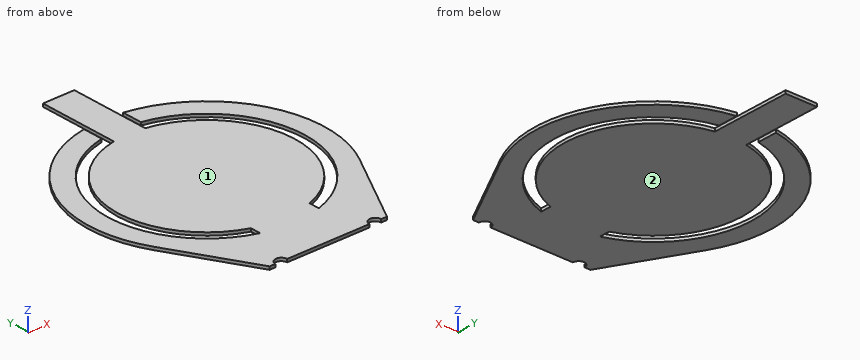
```python
from build123d import *

# Parameters (mm, degrees)
BOSS_EXTRUDE1_DEPTH      = 0.75438
CORTE_EXTRUS_O1_START    = -10
CORTE_EXTRUS_O1_DEPTH    = 10
RESSALTO_EXTRUS_O1_START = -0.75438
RESSALTO_EXTRUS_O1_DEPTH = 0.75438
CORTE_EXTRUS_O2_DEPTH    = 10


with BuildPart() as part:
    # Sketch1 → Boss-Extrude1 (new body)
    with BuildSketch(Plane.XY):
        with BuildLine():
            Line((-15, -35), (15, -35))
            Line((15, -35), (26.292884648, -14.44590658))
            ThreePointArc((26.292884648, -14.44590658), (0, 30), (-26.292884648, -14.44590658))
            Line((-26.292884648, -14.44590658), (-15, -35))
        make_face()
        with BuildLine():
            Line((-7.5, -23.848480035), (-7.5, -21.213203436))
            ThreePointArc((-7.5, -21.213203436), (0, 22.5), (7.5, -21.213203436))
            Line((7.5, -21.213203436), (7.5, -23.848480035))
            ThreePointArc((7.5, -23.848480035), (0, 25), (-7.5, -23.848480035))
        make_face(mode=Mode.SUBTRACT)
    extrude(amount=BOSS_EXTRUDE1_DEPTH)

    # Esboço1 → Corte-extrusão1 (cut)
    with BuildSketch(Plane.XY.offset(0.75438).offset(CORTE_EXTRUS_O1_START)):
        with BuildLine():
            ThreePointArc((-5, 29.580398915), (-2.508787808, 29.894915684), (0, 30))
            ThreePointArc((0, 30), (2.508787808, 29.894915684), (5, 29.580398915))
            Line((5, 29.580398915), (5, 30.901392532))
            Line((5, 30.901392532), (-5, 30.901392532))
            Line((-5, 30.901392532), (-5, 29.580398915))
        make_face()
        with BuildLine():
            Line((0, 27.5), (0, 30))
            ThreePointArc((0, 30), (-2.508787808, 29.894915684), (-5, 29.580398915))
            Line((-5, 29.580398915), (-5, 27.5))
            Line((-5, 27.5), (0, 27.5))
        make_face()
        with BuildLine():
            ThreePointArc((5, 29.580398915), (2.508787808, 29.894915684), (0, 30))
            Line((0, 30), (0, 27.5))
            Line((0, 27.5), (5, 27.5))
            Line((5, 27.5), (5, 29.580398915))
        make_face()
        with BuildLine():
            Line((5, 27.5), (0, 27.5))
            Line((0, 27.5), (0, 25))
            ThreePointArc((0, 25), (2.51272405, 24.873403825), (5, 24.494897428))
            Line((5, 24.494897428), (5, 27.5))
        make_face()
        with BuildLine():
            Line((0, 25), (0, 27.5))
            Line((0, 27.5), (-5, 27.5))
            Line((-5, 27.5), (-5, 24.494897428))
            ThreePointArc((-5, 24.494897428), (-2.51272405, 24.873403825), (0, 25))
        make_face()
        with BuildLine():
            ThreePointArc((5, 24.494897428), (2.51272405, 24.873403825), (0, 25))
            ThreePointArc((0, 25), (-2.51272405, 24.873403825), (-5, 24.494897428))
            Line((-5, 24.494897428), (-5, 24.098607468))
            Line((-5, 24.098607468), (5, 24.098607468))
            Line((5, 24.098607468), (5, 24.494897428))
        make_face()
    extrude(amount=CORTE_EXTRUS_O1_DEPTH, mode=Mode.SUBTRACT)

    # Esboço3 → Ressalto-extrusão1 (add)
    with BuildSketch(Plane.XY.offset(0.75438).offset(RESSALTO_EXTRUS_O1_START)):
        with BuildLine():
            ThreePointArc((-4, 22.141589825), (-2.008012566, 22.410218329), (0, 22.5))
            Line((0, 22.5), (0, 42.5))
            Line((0, 42.5), (-4, 42.5))
            Line((-4, 42.5), (-4, 24.494897428))
            Line((-4, 24.494897428), (-4, 22.141589825))
        make_face()
        with BuildLine():
            Line((0, 42.5), (0, 22.5))
            ThreePointArc((0, 22.5), (2.008012566, 22.410218329), (4, 22.141589825))
            Line((4, 22.141589825), (4, 42.5))
            Line((4, 42.5), (0, 42.5))
        make_face()
    extrude(amount=RESSALTO_EXTRUS_O1_DEPTH)

    # Esboço4 → Corte-extrusão2 (cut)
    with BuildSketch(Plane.XY.offset(0.75438)):
        with BuildLine():
            ThreePointArc((-10.5, -35), (-12, -33.5), (-13.5, -35))
            Line((-13.5, -35), (-12, -35))
            Line((-12, -35), (-10.5, -35))
        make_face()
        with BuildLine():
            Line((-12, -35), (-13.5, -35))
            ThreePointArc((-13.5, -35), (-12, -36.5), (-10.5, -35))
            Line((-10.5, -35), (-12, -35))
        make_face()
        with BuildLine():
            ThreePointArc((13.5, -35), (12, -33.5), (10.5, -35))
            Line((10.5, -35), (13.5, -35))
        make_face()
        with BuildLine():
            Line((13.5, -35), (10.5, -35))
            ThreePointArc((10.5, -35), (12, -36.5), (13.5, -35))
        make_face()
    extrude(amount=-CORTE_EXTRUS_O2_DEPTH, mode=Mode.SUBTRACT)


solid = part.part
```
For this review, take the finished solid that the model builds, in its own axes (mm). Face numbers are marked on the shaded views. Coordinates: 2 decimals unless noted, no trailing zeros. Write each loop counter-clockwise with the first axis right and the second up, starting at its lowest first coordinate (ties: lowest second). Pieces come first, ordered by that corner, then holes. Notation, with made-up numbers: (49.25, -1.75) -> (97.25, -1.75) arc R25 ccw to (97.25, 31.25) -> close; hole circle Ø11 at (31, 46). An arc over 180 degrees is marked (long way). Put each result on its own line as item: value.
Q1. Take a section at B-B, the plane x = 19.5. State the section outline as (y, z) points, then the cut area to 3 significant figures.
From the geometry:
outline: (-26.81, 0) -> (-15.64, 0) -> (-15.64, 0.75) -> (-26.81, 0.75) -> close; (-11.22, 0) -> (11.22, 0) -> (11.22, 0.75) -> (-11.22, 0.75) -> close; (15.64, 0) -> (22.8, 0) -> (22.8, 0.75) -> (15.64, 0.75) -> close
area: 30.8 mm2
Q2. Wall thickness on L1, parallel to X at y = 0, z = 0.1; L2, parallel to Y at x = 15.5, z = 0.5; L3, parallel to X at y = -15.5, z = 0.7: over which ranges is each line inside the solid? List them lowest first.
From the geometry:
L1: x = -30 to -25, -22.5 to 22.5, 25 to 30
L2: y = -34.09 to -19.62, -16.31 to 16.31, 19.62 to 25.69
L3: x = -25.71 to -19.62, -16.31 to 16.31, 19.62 to 25.71
Q3. Clearance check with a flat-ended pin moving along its axis: pin 1 Ø4 at (x, y) = (7.5, 5) entering from -Z. State where the tip first meets the part, or that it passes through.
From the geometry:
pin 1: stops at z = 0
Q4. The part is to be moulded in two halves that separate along Z. For the marked faces 1 and 2, say which applies: +Z half, -Z half, draft (parallel to the pull), parting line (faces both ways), or undercut.
From the geometry:
face 1: +Z half
face 2: -Z half
Q5. Take a section at C-C, the plane z = 0.55. State the section outline as (x, y) points.
From the geometry:
outline: (-26.29, -14.45) -> (-15, -35) -> (-13.5, -35) arc R1.5 cw to (-10.5, -35) -> (10.5, -35) arc R1.5 cw to (13.5, -35) -> (15, -35) -> (26.29, -14.45) arc R30 ccw to (5, 29.58) -> (5, 24.49) arc R25 cw to (7.5, -23.85) -> (7.5, -21.21) arc R22.5 ccw to (4, 22.14) -> (4, 42.5) -> (-4, 42.5) -> (-4, 22.14) arc R22.5 ccw to (-7.5, -21.21) -> (-7.5, -23.85) arc R25 cw to (-5, 24.49) -> (-5, 29.58) arc R30 ccw to start
Q6. Take a section at A-A, the plane y = 27. State the section outline as (x, z) points, then the cut area to 3 significant figures.
From the geometry:
outline: (-13.08, 0) -> (-5, 0) -> (-5, 0.75) -> (-13.08, 0.75) -> close; (-4, 0) -> (4, 0) -> (4, 0.75) -> (-4, 0.75) -> close; (5, 0) -> (13.08, 0) -> (13.08, 0.75) -> (5, 0.75) -> close
area: 18.2 mm2
